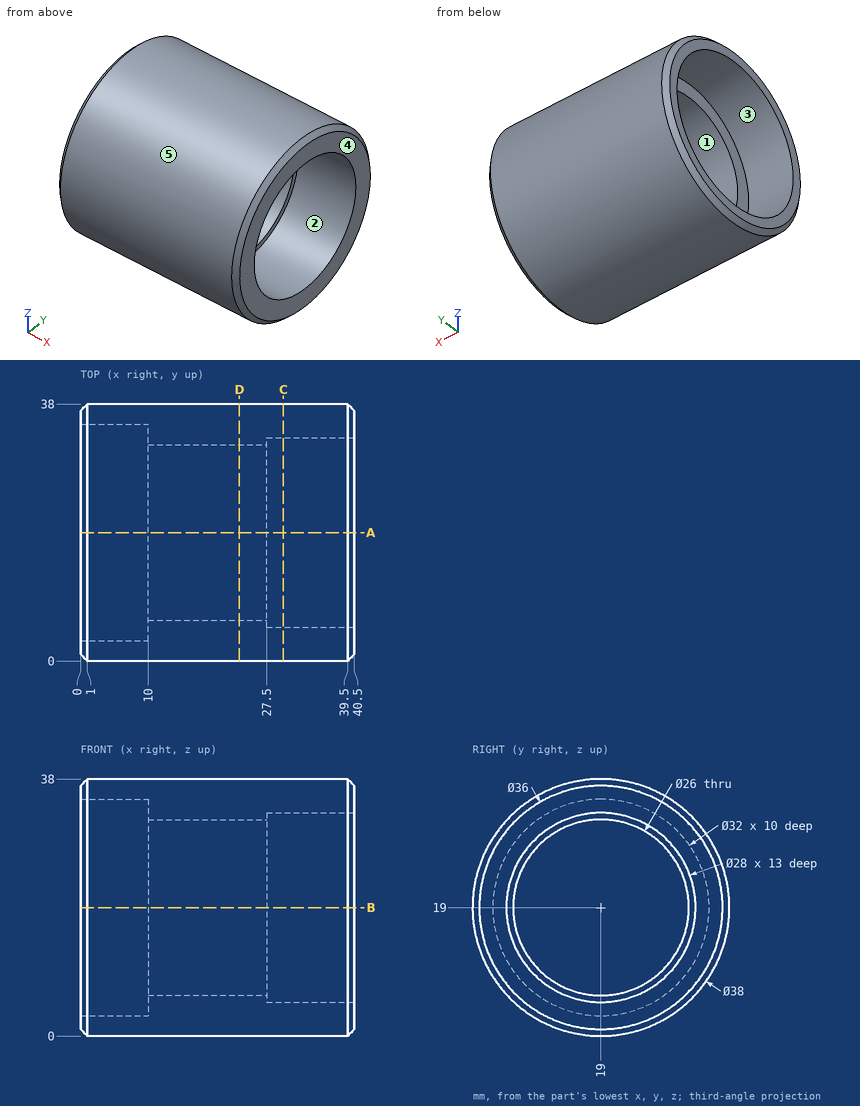
Answer from the drawing. Dimensions are ordinates in mm from the lowest x, y and z of the part. A direction names the side the tool comes from. Coordinates: 2 decimals unless noted, no trailing zeros. Loops run counter-clockwise (first coordinate to the right, second up) from the corner with the lowest first, then second, coordinate; pieces in that order, holes last.
Q1. The part is cut by section D-D on x = 23.5. Write down the section's boundary in (y, z).
Q2. Each of these flat-tipped pins is pushed along its axis until it touches: pin 1 Ø5 at (x, y) = (35, 33) entering from +Z; pin 2 Ø4 at (y, z) = (12.5, 26) entering from -X; pin 3 Ø4 at (x, z) = (16.5, 12.5) entering from +Y. Where does it stop, or does it pass through?
Q3. The part is cut by section A-A on y = 19. Write down the section's boundary in (x, z), and give its area (3 significant figures).
Q4. The mould has two halves that part along Z. Classify the marked faces 3, 4 and 5: +Z half, -Z half, draft (parallel to the pull), parting line (faces both ways), or undercut.
Q5. The part is cut by section C-C on x = 30. Write down the section's boundary in (y, z), and give its area (3 significant figures).
Q6. Which of the six approach directions +Z, -Z, +X, -X, +Y, -Y give full straight-line access (tool end or side, diameter ignored) to the marked faces 1 and 2?
Q7. Consider probe 1 along Y at (x, z) = (34, 19); probe 2 along X at (y, z) = (13, 7); probe 3 along X at (y, z) = (9.5, 31). Determine where each line is inside the solid, lowest interval first.
Results below:
1. outline: circle Ø38 at (19, 19); hole circle Ø26 at (19, 19)
2. pin 1: stops at z = 34.12
2. pin 2: passes through
2. pin 3: stops at y = 37.46
3. outline: (0, 1) - (1, 0) - (39.5, 0) - (40.5, 1) - (40.5, 5) - (27.5, 5) - (27.5, 6) - (10, 6) - (10, 3) - (0, 3) - close; (0, 35) - (10, 35) - (10, 32) - (27.5, 32) - (27.5, 33) - (40.5, 33) - (40.5, 37) - (39.5, 38) - (1, 38) - (0, 37) - close
3. area: 398 mm2
4. face 3: undercut
4. face 4: draft
4. face 5: parting line
5. outline: circle Ø38 at (19, 19); hole circle Ø28 at (19, 19)
5. area: 518 mm2
6. face 1: +X, -X
6. face 2: +X
7. probe 1: y = 0 to 5, 33 to 38
7. probe 2: x = 10 to 27.5
7. probe 3: x = 10 to 40.5
